Verification items for the finished model (mm, model axes). Coordinates: 2 decimals unless noted, no trailing zeros. Order: outer loops, then holes, each group sorted by start corner. A loop starts at its lowest first (then second) coordinate and runs counter-clockwise, first axis right, second up. Notation, with made-up numbers: M -25.75,13 L -5.75,13 A20 cw -5.75,41 Z; hole C -39.5,61 d5. An arc over 180 degrees is marked long. Use one line per item in the form item = value. Start each with the question number.
```python
from build123d import *

# Parameters (mm, degrees)
SKETCH_R    = 4
SKETCH_R_2  = 5
PAD_DEPTH   = 5
FILLET_R    = 0.5
FILLET001_R = 0.5


with BuildPart() as part:
    # Sketch → Pad (new body)
    with BuildSketch(Plane.XY):
        with BuildLine():
            Line((-25, 40), (25, 40))
            ThreePointArc((35, 30), (32.071068, 37.071068), (25, 40))
            Line((35, 30), (35, 22))
            ThreePointArc((35, 22), (37.343146, 16.343146), (43, 14))
            Line((43, 14), (55, 14))
            Line((55, 14), (55, -11))
            Line((55, -11), (15, -36))
            Line((15, -36), (-15, -36))
            Line((-15, -36), (-55, -11))
            Line((-55, -11), (-55, 14))
            Line((-55, 14), (-43, 14))
            ThreePointArc((-43, 14), (-37.343146, 16.343146), (-35, 22))
            Line((-35, 22), (-35, 30))
            ThreePointArc((-25, 40), (-32.071068, 37.071068), (-35, 30))
        make_face()
        with Locations((0, -28)):
            Circle(SKETCH_R, mode=Mode.SUBTRACT)
        with Locations((45, 0)):
            Circle(SKETCH_R, mode=Mode.SUBTRACT)
        with Locations((-45, 0)):
            Circle(SKETCH_R, mode=Mode.SUBTRACT)
        with Locations((25, 30)):
            Circle(SKETCH_R_2, mode=Mode.SUBTRACT)
        with Locations((-25, 30)):
            Circle(SKETCH_R_2, mode=Mode.SUBTRACT)
        with BuildLine():
            ThreePointArc((-4, 14.456832), (0, -15), (4, 14.456832))
            Line((4, 25), (4, 14.456832))
            ThreePointArc((4, 25), (0, 29), (-4, 25))
            Line((-4, 25), (-4, 14.456832))
        make_face(mode=Mode.SUBTRACT)
    extrude(amount=PAD_DEPTH)

    # Fillet
    fillet_edges = [part.edges().sort_by_distance(p)[0] for p in [
        (-55, 1.5, 5),
        (-35, -23.5, 5),
        (0, -36, 5),
        (35, -23.5, 5),
        (55, 1.5, 5),
        (49, 14, 5),
        (37.343146, 16.343146, 5),
        (35, 26, 5),
        (32.071068, 37.071068, 5),
        (0, 40, 5),
        (-32.071068, 37.071068, 5),
        (-35, 26, 5),
        (-37.343146, 16.343146, 5),
        (-49, 14, 5),
    ]]
    fillet(fillet_edges, radius=FILLET_R)

    # Fillet001
    fillet001_edges = [part.edges().sort_by_distance(p)[0] for p in [
        (0, -36, 0),
        (-35, -23.5, 0),
        (-55, 1.5, 0),
        (-49, 14, 0),
        (-37.343146, 16.343146, 0),
        (-35, 26, 0),
        (-32.071068, 37.071068, 0),
        (0, 40, 0),
        (32.071068, 37.071068, 0),
        (35, 26, 0),
        (37.343146, 16.343146, 0),
        (49, 14, 0),
        (55, 1.5, 0),
        (35, -23.5, 0),
    ]]
    fillet(fillet001_edges, radius=FILLET001_R)


solid = part.part
```
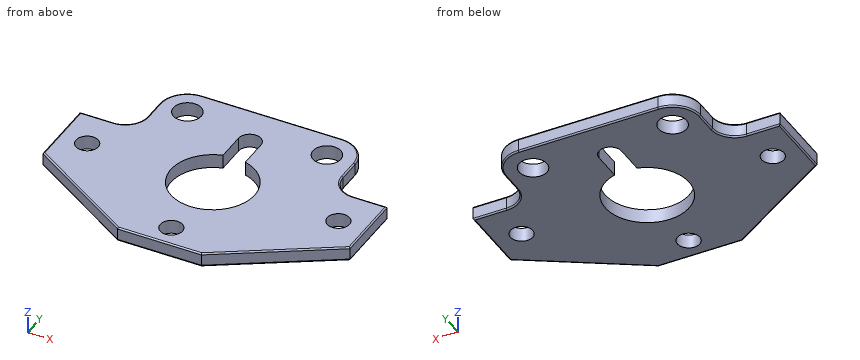
1. Cross-section at D-D on y = 8.5. Enter the section's corners in (x, z), and give its area (3 significant figures).
2. Depth check by flat-ended pin: P1, Ø1.5, axis at x = -34.5, z = 2, coming from the +Y side; P2, Ø8, axis at x = -25, y = 30, coming from the +Z side; P3, Ø2.5, axis at y = 20, z = 2.5, coming from the -X side; P4, Ø2, axis at y = 25.5, z = 2.5, coming from the +X side. Enter the tip coordinate at first touch or a pass-through.
3. Cross-section at A-A on y = 0. Enter the section's corners in (x, z), and give its area (3 significant figures).
4. Material ranges on line 1 along X through (y, z) = (10.5, 0.4); line 2 along Y through (x, z) = (-10, 0.85); line 3 along Y through (x, z) = (-25, 2.55), recorded low to high.
5. Cross-section at C-C on z = 3.05. Enter the section's corners in (x, y).
6. Cross-section at B-B on x = 0. Enter the section's corners in (y, z).
Final values:
q1.outline = M -55,0.5 A0.5 ccw -54.5,0 L -12.36,0 L -12.36,5 L -54.5,5 A0.5 ccw -55,4.5 Z; M 12.36,0 L 54.5,0 A0.5 ccw 55,0.5 L 55,4.5 A0.5 ccw 54.5,5 L 12.36,5 Z
q1.area = 426 mm2
q2.P1 = 34.84
q2.P2 = through
q2.P3 = -35.69
q2.P4 = 35
q3.outline = M -55,0.5 A0.5 ccw -54.5,0 L -49,0 L -49,5 L -54.5,5 A0.5 ccw -55,4.5 Z; M -41,0 L -15,0 L -15,5 L -41,5 Z; M 15,0 L 41,0 L 41,5 L 15,5 Z; M 49,0 L 54.5,0 A0.5 ccw 55,0.5 L 55,4.5 A0.5 ccw 54.5,5 L 49,5 Z
q3.area = 320 mm2
q4.line_1 = -54.99 to -10.71, 10.71 to 54.99
q4.line_2 = -36 to -11.18, 11.18 to 40
q4.line_3 = -29.75 to 25, 35 to 40
q5.outline = M -55,-11 L -15,-36 L 15,-36 L 55,-11 L 55,14 L 43,14 A8 cw 35,22 L 35,30 A10 ccw 25,40 L -25,40 A10 ccw -35,30 L -35,22 A8 cw -43,14 L -55,14 Z; hole C -45,0 d8; hole C -25,30 d10; hole C 0,-28 d8; hole M -4,14.46 A15 ccw long 4,14.46 L 4,25 A4 ccw -4,25 Z; hole C 25,30 d10; hole C 45,0 d8
q6.outline = M -36,0.5 A0.5 ccw -35.5,0 L -32,0 L -32,5 L -35.5,5 A0.5 ccw -36,4.5 Z; M -24,0 L -15,0 L -15,5 L -24,5 Z; M 29,0 L 39.5,0 A0.5 ccw 40,0.5 L 40,4.5 A0.5 ccw 39.5,5 L 29,5 Z
